Could you check a few things on this model? Use its own coordinates, in mm. Face numbers are marked on the shaded views. A direction names the side the tool comes from. Give positions to 0.01 mm unless a question says otherwise; leave off trailing zeros. Order: outer loops, then holes, each group sorted by start corner. A loop starts at its lowest first (then second) coordinate and runs counter-clockwise, first axis right, second up.
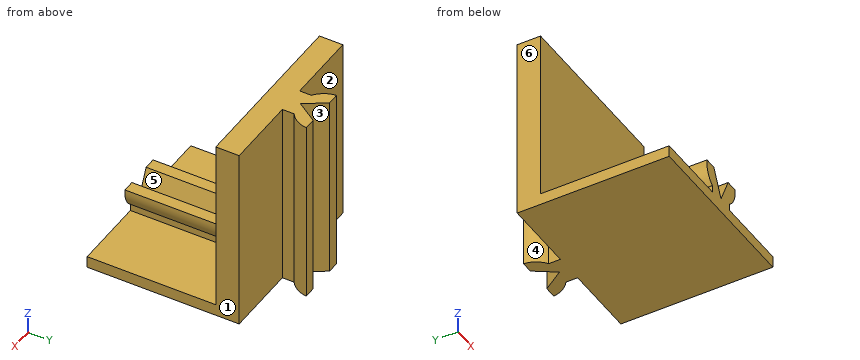
from build123d import *

# Parameters (mm, degrees)
SKETCH_W     = 15
SKETCH_H     = 13
PAD_DEPTH    = 1
SKETCH001_W  = 15
SKETCH001_H  = 2
PAD001_DEPTH = 15
PAD002_DEPTH = 11
PAD003_DEPTH = 16


with BuildPart() as part:
    # Sketch → Pad (new body)
    with BuildSketch(Plane.XY):
        Rectangle(SKETCH_W, SKETCH_H)
    extrude(amount=PAD_DEPTH)

    # Sketch001 → Pad001 (new body)
    with BuildSketch(Plane.XY.offset(1)):
        with Locations((0, 5.5)):
            Rectangle(SKETCH001_W, SKETCH001_H)
    extrude(amount=PAD001_DEPTH)

    # Sketch002 → Pad002 (new body)
    with BuildSketch(Plane.XZ.offset(6.5)):
        with BuildLine():
            Line((-1.25, 1), (1.25, 1))
            Line((1.25, 1), (1.25, 1.6))
            ThreePointArc((1.25, 1.6), (1.895909, 2.445045), (2.031445, 3.5))
            Line((2.031445, 3.5), (1.031445, 3.5))
            Line((1.031445, 3.5), (0, 1.224808))
            Line((0, 1.224808), (-1.031445, 3.5))
            Line((-2.031445, 3.5), (-1.031445, 3.5))
            ThreePointArc((-2.031445, 3.5), (-1.895909, 2.445045), (-1.25, 1.6))
            Line((-1.25, 1), (-1.25, 1.6))
        make_face()
    extrude(amount=-PAD002_DEPTH)

    # Sketch003 → Pad003 (new body)
    with BuildSketch(Plane.XY.offset(16)):
        with BuildLine():
            Line((-1.25, 7.5), (-1.25, 6.5))
            Line((-1.25, 6.5), (1.25, 6.5))
            Line((1.25, 6.5), (1.25, 7.5))
            ThreePointArc((1.25, 7.5), (1.896907, 8.196052), (2.189917, 9.1))
            Line((2.189917, 9.1), (1.189917, 9.1))
            Line((1.189917, 9.1), (0, 7.310387))
            Line((0, 7.310387), (-1.189917, 9.1))
            Line((-2.189917, 9.1), (-1.189917, 9.1))
            ThreePointArc((-2.189917, 9.1), (-1.896907, 8.196052), (-1.25, 7.5))
        make_face()
    extrude(amount=-PAD003_DEPTH)


solid = part.part
Item 1: For pin 1 (1 mm diameter, centred on x = 1, z = 12, fed in from -Y); pin 2 (2 mm diameter, centred on x = 6, y = 0.5, fed in from +Z); pin 3 (0.8 mm diameter, centred on x = 1.5, y = 0, fed in from +Z), each with a flat end and sliding along its axis, tell me the tip position at first contact or that it passes through.
Findings:
pin 1: stops at y = 4.5
pin 2: stops at z = 1
pin 3: stops at z = 3.5
Item 2: Imagine slicing it at A-A on x = 1.75. List the corners of the cut face in (y, z) for me.
Findings:
outline: (-6.5, 0) - (6.5, 0) - (6.5, 16) - (4.5, 16) - (4.5, 3.5) - (-6.5, 3.5) - (-6.5, 2.16) - (4.5, 2.16) - (4.5, 1) - (-6.5, 1) - close; (7.98, 0) - (9.1, 0) - (9.1, 16) - (7.98, 16) - close
Item 3: Imagine slicing it at D-D on x = 4.5. List the corners of the cut face in (y, z) for me.
Findings:
outline: (-6.5, 0) - (6.5, 0) - (6.5, 16) - (4.5, 16) - (4.5, 1) - (-6.5, 1) - close
Item 4: We'd pull the mould along X, two halves only. Please class the marked faces 1, 2, 3 and 4: +X half, -X half, draft (parallel to the pull), parting line (faces both ways), or undercut.
Findings:
face 1: +X half
face 2: draft
face 3: undercut
face 4: -X half
Item 5: Imagine slicing it at B-B on y = -4.5. List the corners of the cut face in (x, z) for me.
Findings:
outline: (-7.5, 0) - (7.5, 0) - (7.5, 1) - (1.25, 1) - (1.25, 1.6) arc R2.05 ccw to (2.03, 3.5) - (1.03, 3.5) - (0, 1.22) - (-1.03, 3.5) - (-2.03, 3.5) arc R2.05 ccw to (-1.25, 1.6) - (-1.25, 1) - (-7.5, 1) - close
Item 6: For the marked faces 5 and 6, which set-ups out of +Z, -Z, +X, -X, +Y, -Y let a thin tool reach every point of the face, with its end or its side?
Findings:
face 5: +Z, -Y
face 6: +Z, -Z, -X, +Y, -Y
Item 7: Please list where these lines run through material, in increasing order: line 1 along Y through (x, z) = (2.75, 2.25); line 2 along Z through (x, y) = (2.75, -0.75); line 3 along Y through (x, z) = (-2, 14.75).
Findings:
line 1: y = 4.5 to 6.5
line 2: z = 0 to 1
line 3: y = 4.5 to 6.5, 8.39 to 9.1
Item 8: Imagine slicing it at C-C on z = 9.25. List the corners of the cut face in (x, y) for me.
Findings:
outline: (-7.5, 4.5) - (7.5, 4.5) - (7.5, 6.5) - (1.25, 6.5) - (1.25, 7.5) arc R2.2 ccw to (2.19, 9.1) - (1.19, 9.1) - (0, 7.31) - (-1.19, 9.1) - (-2.19, 9.1) arc R2.2 ccw to (-1.25, 7.5) - (-1.25, 6.5) - (-7.5, 6.5) - close
